Check sheet for the modelled part. Datum: model origin and axes. Units: mm. Face numbers are marked on the shaded views. A direction names the side the tool comes from. Give positions to 0.01 mm unless a question says otherwise; leave off trailing zeros. Write each loop counter-clockwise with the first axis right and the second up, starting at its lowest first coordinate (ties: lowest second). Pieces come first, ordered by that corner, then holes. Notation, with made-up numbers: (30, 67.25) -> (46, 67.25) arc R19 ccw to (46, 94.25) -> close; hole circle Ø7 at (-8, -23.75). An arc over 180 degrees is marked (long way). Return JSON: item names as keys, results as strings.
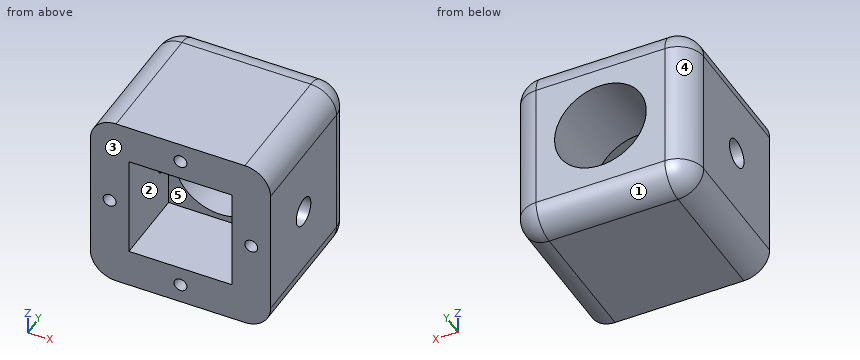
from build123d import *

# Parameters (mm, degrees)
SKETCH1_W                      = 35
SKETCH1_H                      = 35
BOSS_EXTRUDE1_DEPTH            = 30
SKETCH2_W                      = 20
SKETCH2_H                      = 20
CUT_EXTRUDE1_DEPTH             = 15
SKETCH3_R                      = 8.9
CUT_EXTRUDE2_DEPTH             = 58.879184514
CBORE_FOR_M2_SHCS1_D           = 2.6
CBORE_FOR_M2_SHCS1_DEPTH       = 7.5
CBORE_FOR_M2_SHCS1_CBORE_D     = 5.5
CBORE_FOR_M2_SHCS1_CBORE_DEPTH = 6
CBORE_FOR_M2_SHCS2_D           = 2.6
CBORE_FOR_M2_SHCS2_CBORE_D     = 5.5
CBORE_FOR_M2_SHCS2_CBORE_DEPTH = 6
FILLET1_R                      = 5
FILLET2_R                      = 5
M3X0_5_TAPPED_HOLE1_D          = 2.5
M3X0_5_TAPPED_HOLE1_DEPTH      = 5
M3X0_5_TAPPED_HOLE1_TIP        = 0.751075774


with BuildPart() as part:
    # Sketch1 → Boss-Extrude1 (new body)
    with BuildSketch(Plane(origin=(0, 0, 0), x_dir=(1, 0, 0), z_dir=(0, 1, 0))):
        with Locations((17.5, 17.5)):
            Rectangle(SKETCH1_W, SKETCH1_H)
    extrude(amount=BOSS_EXTRUDE1_DEPTH)

    # Sketch2 → Cut-Extrude1 (cut)
    with BuildSketch(Plane.XZ):
        with Locations((17.5, -17.5)):
            Rectangle(SKETCH2_W, SKETCH2_H)
    extrude(amount=-CUT_EXTRUDE1_DEPTH, mode=Mode.SUBTRACT)

    # Sketch3 → Cut-Extrude2 (cut, through all)
    with BuildSketch(Plane(origin=(0, 30, 0), x_dir=(1, 0, 0), z_dir=(0, 1, 0))):
        with Locations(Location((17.5, 17.5, 0), (0, 0, 270))):
            Circle(SKETCH3_R)
    extrude(amount=-CUT_EXTRUDE2_DEPTH, mode=Mode.SUBTRACT)

    # CBORE for M2 SHCS1
    with Locations(Plane(origin=(35, 12.5, -17.5), x_dir=(0, 0, 1), z_dir=(1, 0, 0))):
        with Locations((0, 0)):
            CounterBoreHole(CBORE_FOR_M2_SHCS1_D / 2, CBORE_FOR_M2_SHCS1_CBORE_D / 2, CBORE_FOR_M2_SHCS1_CBORE_DEPTH, depth=CBORE_FOR_M2_SHCS1_DEPTH)

    # CBORE for M2 SHCS2 (through all)
    with Locations(Plane(origin=(0, 12.5, -17.5), x_dir=(0, 0, -1), z_dir=(-1, 0, 0))):
        with Locations((0, 0)):
            CounterBoreHole(CBORE_FOR_M2_SHCS2_D / 2, CBORE_FOR_M2_SHCS2_CBORE_D / 2, CBORE_FOR_M2_SHCS2_CBORE_DEPTH)

    # Fillet1
    fillet1_edges = [part.edges().sort_by_distance(p)[0] for p in [
        (35, 30, -17.5),
        (17.5, 30, -35),
        (0, 30, -17.5),
        (17.5, 30, 0),
    ]]
    fillet(fillet1_edges, radius=FILLET1_R)

    # Fillet2
    # the kernel refuses this fillet: 5 mm, written as the material it takes off along each edge
    with BuildSketch(Plane(origin=(30, 25, -30), x_dir=(0, 0, -1), z_dir=(1, 0, 0))) as fillet2_piece_1_section:
        Polygon((0, 0), (FILLET2_R, 0), (FILLET2_R, FILLET2_R), (0, FILLET2_R), align=None)
    fillet2_piece_1 = extrude(amount=FILLET2_R, mode=Mode.PRIVATE)
    fillet2_piece_1 = fillet2_piece_1 - Plane(origin=(30, 25, -30), x_dir=(0, -0.7071067811865475, 0.7071067811865475), z_dir=(1, 0, 0)) * Sphere(FILLET2_R, mode=Mode.PRIVATE)
    add(fillet2_piece_1, mode=Mode.SUBTRACT)
    with BuildSketch(Plane(origin=(30, 25, -5), x_dir=(1, 0, 0), z_dir=(0, 0, 1))) as fillet2_piece_2_section:
        Polygon((0, 0), (FILLET2_R, 0), (FILLET2_R, FILLET2_R), (0, FILLET2_R), align=None)
    fillet2_piece_2 = extrude(amount=FILLET2_R, mode=Mode.PRIVATE)
    fillet2_piece_2 = fillet2_piece_2 - Plane(origin=(30, 25, -5), x_dir=(-0.7071067811865475, -0.7071067811865475, 0), z_dir=(0, 0, 1)) * Sphere(FILLET2_R, mode=Mode.PRIVATE)
    add(fillet2_piece_2, mode=Mode.SUBTRACT)
    with BuildSketch(Plane(origin=(5, 25, -30), x_dir=(0, 0, -1), z_dir=(-1, 0, 0))) as fillet2_piece_3_section:
        Polygon((0, 0), (FILLET2_R, 0), (FILLET2_R, -FILLET2_R), (0, -FILLET2_R), align=None)
    fillet2_piece_3 = extrude(amount=FILLET2_R, mode=Mode.PRIVATE)
    fillet2_piece_3 = fillet2_piece_3 - Plane(origin=(5, 25, -30), x_dir=(0, -0.7071067811865475, 0.7071067811865475), z_dir=(-1, 0, 0)) * Sphere(FILLET2_R, mode=Mode.PRIVATE)
    add(fillet2_piece_3, mode=Mode.SUBTRACT)
    with BuildSketch(Plane(origin=(5, 25, -5), x_dir=(-1, 0, 0), z_dir=(0, 0, 1))) as fillet2_piece_4_section:
        Polygon((0, 0), (FILLET2_R, 0), (FILLET2_R, -FILLET2_R), (0, -FILLET2_R), align=None)
    fillet2_piece_4 = extrude(amount=FILLET2_R, mode=Mode.PRIVATE)
    fillet2_piece_4 = fillet2_piece_4 - Plane(origin=(5, 25, -5), x_dir=(0.7071067811865475, -0.7071067811865475, 0), z_dir=(0, 0, 1)) * Sphere(FILLET2_R, mode=Mode.PRIVATE)
    add(fillet2_piece_4, mode=Mode.SUBTRACT)
    with BuildSketch(Plane(origin=(0, -12.5, 0), x_dir=(1, 0, 0), z_dir=(0, 1, 0)), Plane(origin=(0, -12.5, -35), x_dir=(0, 0, 1), z_dir=(0, 1, 0))) as fillet2_piece_5:
        with BuildLine():
            CenterArc((FILLET2_R, FILLET2_R), FILLET2_R, 180, 90)
            Line((0, FILLET2_R), (0, 0))
            Line((0, 0), (FILLET2_R, 0))
        make_face()
    extrude(amount=37.5, mode=Mode.SUBTRACT)
    with BuildSketch(Plane(origin=(35, -12.5, -35), x_dir=(0, 0, 1), z_dir=(0, 1, 0)), Plane(origin=(35, -12.5, 0), x_dir=(-1, 0, 0), z_dir=(0, 1, 0))) as fillet2_piece_6:
        with BuildLine():
            CenterArc((FILLET2_R, -FILLET2_R), FILLET2_R, 90, 90)
            Line((0, -FILLET2_R), (0, 0))
            Line((0, 0), (FILLET2_R, 0))
        make_face()
    extrude(amount=37.5, mode=Mode.SUBTRACT)

    # M3x0.5 Tapped Hole1
    with Locations(Plane(origin=(17.5, 0, -31.25), x_dir=(0, 0, -1), z_dir=(0, -1, 0))):
        with Locations((0, 0), (-13.75, -13.75), (-27.5, 0), (-13.75, 13.75)):
            Hole(M3X0_5_TAPPED_HOLE1_D / 2, depth=M3X0_5_TAPPED_HOLE1_DEPTH)
            with Locations((0, 0, -(M3X0_5_TAPPED_HOLE1_DEPTH + M3X0_5_TAPPED_HOLE1_TIP / 2))):  # 118° drill point
                Cone(0, M3X0_5_TAPPED_HOLE1_D / 2, M3X0_5_TAPPED_HOLE1_TIP, mode=Mode.SUBTRACT)


solid = part.part
(1) Release check for a two-part mould opening along Z. For the marked faces 1, 2 and 3 record: pulls with the +Z half, pulls with the -Z half, needs draft (parallel to the pull), parting line crosses it, or undercut.
Reply:
{"face 1": "pulls with the -Z half", "face 2": "undercut", "face 3": "needs draft"}
(2) Cross-section at C-C on z = -22. Enter the section's corners in (x, y).
Reply:
{"outline": "(0, 0) -> (7.5, 0) -> (7.5, 15) -> (9.82, 15) -> (9.82, 30) -> (5, 30) arc R5 ccw to (0, 25) -> close; (25.18, 15) -> (27.5, 15) -> (27.5, 0) -> (35, 0) -> (35, 25) arc R5 ccw to (30, 30) -> (25.18, 30) -> close"}
(3) Thickness scan on L1, parallel to Z at x = 19.5, y = 1.5; L2, parallel to X at y = 3.85, z = -17.5; L3, parallel to X at y = 11, z = -22.5. Record the ranges inside material, lowest first.
Reply:
{"L1": "-35 to -27.5, -7.5 to 0", "L2": "0 to 2.5, 5 to 7.5, 27.5 to 30, 32.5 to 35", "L3": "0 to 7.5, 27.5 to 35"}
(4) Set-up check for the marked faces 4 and 5: record each of +Z, -Z, +X, -X, +Y, -Y from which the full face is reachable in a straight line by a thin tool's end or side.
Reply:
{"face 4": "+Z, -Z, -X, +Y", "face 5": "-Y"}
(5) Cross-section at D-D on y = 21.5. Enter the section's corners in (x, z).
Reply:
{"outline": "(0, -30) arc R5 ccw to (5, -35) -> (30, -35) arc R5 ccw to (35, -30) -> (35, -5) arc R5 ccw to (30, 0) -> (5, 0) arc R5 ccw to (0, -5) -> close; hole circle Ø17.8 at (17.5, -17.5)"}
(6) Cross-section at A-A on y = 12.5. Enter the section's corners in (x, z).
Reply:
{"outline": "(0, -30) arc R5 ccw to (5, -35) -> (30, -35) arc R5 ccw to (35, -30) -> (35, -20.25) -> (29, -20.25) -> (29, -18.8) -> (27.5, -18.8) -> (27.5, -27.5) -> (7.5, -27.5) -> (7.5, -18.8) -> (6, -18.8) -> (6, -20.25) -> (0, -20.25) -> close; (0, -14.75) -> (6, -14.75) -> (6, -16.2) -> (7.5, -16.2) -> (7.5, -7.5) -> (27.5, -7.5) -> (27.5, -16.2) -> (29, -16.2) -> (29, -14.75) -> (35, -14.75) -> (35, -5) arc R5 ccw to (30, 0) -> (5, 0) arc R5 ccw to (0, -5) -> close"}
(7) Cross-section at B-B on x = 28. Enter the section's corners in (y, z).
Reply:
{"outline": "(0, -35) -> (25, -35) arc R5 ccw to (30, -30) -> (30, -5) arc R5 ccw to (25, 0) -> (0, 0) -> close; hole circle Ø2.6 at (12.5, -17.5)"}
(8) Depth check by flat-ended pin: pin 1 Ø6 at (x, z) = (21, -16) entering from -Y; pin 2 Ø2 at (x, z) = (17.5, -31.25) entering from -Y; pin 3 Ø3 at (y, z) = (12.5, -17.5) entering from -X; pin 4 Ø2 at (x, z) = (3.75, -17.5) entering from +Y. Enter the tip coordinate at first touch or a pass-through.
Reply:
{"pin 1": "through", "pin 2": "y = 5.15", "pin 3": "x = 6", "pin 4": "y = 29.99"}
